Geometry check sheet. Reference: the model listing, model coordinates, mm. Face numbers are marked on the shaded views. A direction names the side the tool comes from. Round coordinates to 2 decimals unless told otherwise and drop trailing zeros. Order: outer loops, then holes, each group sorted by start corner. A loop starts at its lowest first (then second) coordinate and runs counter-clockwise, first axis right, second up. Notation, with made-up numbers: (9, 60) -> (13, 60) arc R32 cw to (13, 91) -> close; hole circle Ø5 at (66, -32). An arc over 180 degrees is marked (long way). Use a Markdown table: item, result. Add a question column.
Item 1: Sectioned sample at B-B, the plane z = 0. Record the cut outline in (x, y).
Item 2: Sectioned sample at A-A, the plane y = 166. Record the cut outline in (x, z), and give its area (3 significant figures).
Item 3: Mould release check, pull along Z, two halves, no side actions. Record for the marked faces 1, 2 and 3: pulls with the +Z half, pulls with the -Z half, needs draft (parallel to the pull), parting line crosses it, or undercut.
Item 4: Set-up check for the marked faces 4 and 5: record each of +Z, -Z, +X, -X, +Y, -Y from which the full face is reachable in a straight line by a thin tool's end or side.
Item 5: Material ranges on probe 1 along Z at (x, y) = (15, 128); probe 2 along X at (y, z) = (151, -25); probe 3 along Z at (x, y) = (-8.5, 71), recorded low to high. Write a range as [from, to].
Item 6: Gauge pin test, flat ends, axial feed: pin 1 Ø1.5 at (x, y) = (13.5, 93.5) entering from -Z; pin 2 Ø1.5 at (x, z) = (20.5, 0) entering from -Y; pin 3 Ø10 at (x, y) = (-17.5, 55) entering from -Z. Record the tip position at first contact, or that the pin passes through.
Item 7: Sectioned sample at C-C, the plane x = 15. Record the cut outline in (y, z).
Item 8: Sectioned sample at D-D, the plane z = -24.5. Record the cut outline in (x, y), and give its area (3 significant figures).
from build123d import *

# Parameters (mm, degrees)
BOSS_EXTRUDE1_DEPTH = 200
SKETCH2_W           = 9.23188111
SKETCH2_H           = 28.936228776
SKETCH2_W_2         = 10.092838874
CUT_EXTRUDE1_DEPTH  = 6


with BuildPart() as part:
    # Sketch1 → Boss-Extrude1 (new body)
    with BuildSketch(Plane(origin=(0, 0, 0), x_dir=(1, 0, 0), z_dir=(0, 1, 0))):
        with BuildLine():
            Line((22.5, -2.5), (-22.5, -2.5))
            Line((-22.5, -2.5), (-22.5, 2.5))
            Line((-22.5, 2.5), (-12.701705922, 2.5))
            Line((-12.701705922, 2.5), (-5, 15.839745962))
            ThreePointArc((-5, 15.839745962), (0, 34.5), (5, 15.839745962))
            Line((5, 15.839745962), (12.701705922, 2.5))
            Line((12.701705922, 2.5), (22.5, 2.5))
            Line((22.5, 2.5), (22.5, -2.5))
        make_face()
    extrude(amount=BOSS_EXTRUDE1_DEPTH)

    # Sketch2 → Cut-Extrude1 (cut, through all)
    with BuildSketch(Plane(origin=(0, 0, -2.5), x_dir=(-1, 0, 0), z_dir=(0, 0, -1))):
        with Locations((22.5, 11.786741845)):
            Rectangle(SKETCH2_W, SKETCH2_H)
        with Locations((-22.5, 11.786741845)):
            Rectangle(SKETCH2_W_2, SKETCH2_H)
    extrude(amount=-CUT_EXTRUDE1_DEPTH, mode=Mode.SUBTRACT)


solid = part.part
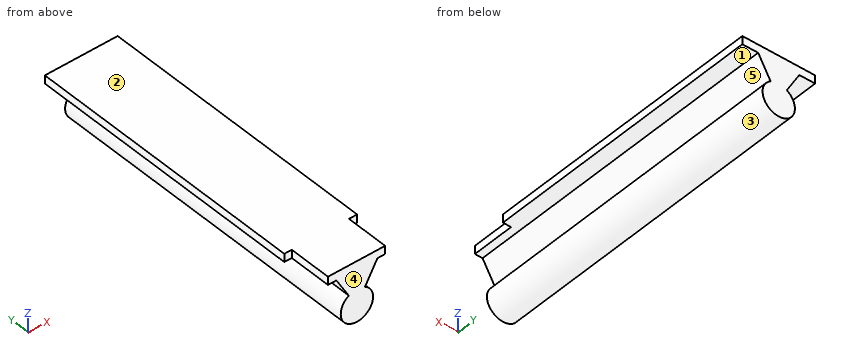
Found:
| question | item | result |
|---|---|---|
| 1 | outline | (-22.5, 26.25) -> (-17.88, 26.25) -> (-17.88, 0) -> (17.45, 0) -> (17.45, 26.25) -> (22.5, 26.25) -> (22.5, 200) -> (-22.5, 200) -> close |
| 2 | outline | (-22.5, -2.5) -> (-12.7, -2.5) -> (-5, -15.84) arc R10 ccw (long way) to (5, -15.84) -> (12.7, -2.5) -> (22.5, -2.5) -> (22.5, 2.5) -> (-22.5, 2.5) -> close |
| 2 | area | 766 mm2 |
| 3 | face 1 | pulls with the -Z half |
| 3 | face 2 | pulls with the +Z half |
| 3 | face 3 | undercut |
| 4 | face 4 | +Z, -Z, +X, -X, -Y |
| 4 | face 5 | +X, +Y, -Y |
| 5 | probe 1 | z = [-2.5, 2.5] |
| 5 | probe 2 | x = [-9.99, 9.99] |
| 5 | probe 3 | z = [-29.77, -19.23], [-9.78, 2.5] |
| 6 | pin 1 | stops at z = -2.5 |
| 6 | pin 2 | stops at y = 26.25 |
| 6 | pin 3 | stops at z = -2.85 |
| 7 | outline | (0, -2.5) -> (200, -2.5) -> (200, 2.5) -> (0, 2.5) -> close |
| 8 | outline | (-10, 0) -> (10, 0) -> (10, 200) -> (-10, 200) -> close |
| 8 | area | 4,000 mm2 |
